Autodesk Fusion 360 part; units mm, degrees
sketch "Control Panel Top" plane through (0, 0, 0) normal (0, 0, 1) x (1, 0, 0)
  line L0 (0, 0) -> (270, 0)
  line L1 (270, 0) -> (270, 86.085)
  line L2 (270, 86.085) -> (0, 86.085)
  line L3 (0, 86.085) -> (0, 0)
  dimension "d6" = 270
  dimension "d7" = 86.085
extrude "Extrude1" add sketch "Control Panel Top" along normal blind 6
sketch "Button Layout" plane through (0, 0, 6) normal (0, 0, 1) x (-1, 0, 0)
  line L0 (0, -86.085) -> (0, 0)
  line L1 (0, 0) -> (-270, 0)
  line L2 (-270, 0) -> (-270, -86.085)
  line L3 (-270, -86.085) -> (0, -86.085)
  circle A0 centre (-90, -43) radius 15
  circle A1 centre (-140, -43) radius 15
  circle A2 centre (-40, -43) radius 15
  dimension "d12" = 30
  dimension "d13" = 30
  dimension "d14" = 30
  dimension "d17" = 40
  dimension "d20" = 50
  dimension "d21" = 43
  dimension "d22" = 43
  dimension "d23" = 43
  dimension "d24" = 50
extrude "Extrude2" cut sketch "Button Layout" against normal blind 6 contours A0 | A1
extrude "Extrude3" cut sketch "Button Layout" against normal blind 6 contours A2
equation "MDFThickness = 6 mm"
equation "d2 = MDFThickness"
equation "controlPanelTopLength = 75 mm"
equation "controlPanelTopWidth = 250 mm"
equation "arcadeButtonDiameter = 30 mm"
equation "d12 = arcadeButtonDiameter"
equation "d13 = arcadeButtonDiameter"
equation "d14 = arcadeButtonDiameter"
equation "d21 = ( 86 / 2 ) * 1 mm"
equation "d22 = ( 86 / 2 ) * 1 mm"
equation "d23 = ( 86 / 2 ) * 1 mm"
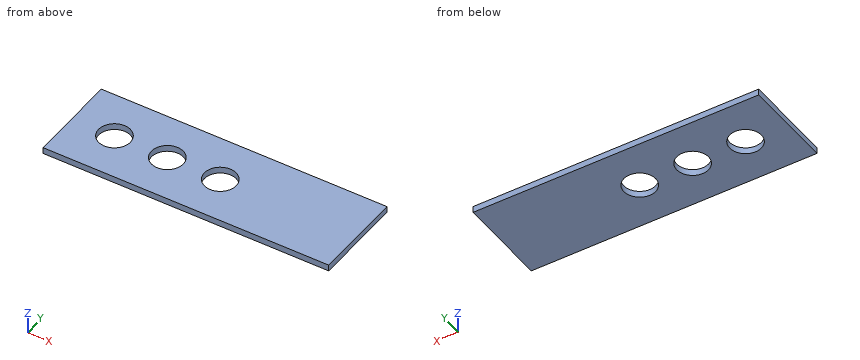
Can you work these out from the model? Positions are in its coordinate system, mm. Coordinates: 2 decimals unless noted, no trailing zeros. Write each loop counter-clockwise with the first axis right and the second up, starting at its lowest first coordinate (ties: lowest second). Pieces come first, ordered by that corner, then holes. Notation, with made-up numbers: (-1.5, -9.75) -> (6.5, -9.75) arc R33 ccw to (6.5, 28.25) -> close; hole circle Ø6 at (26.25, 66.5). An arc over 180 degrees is marked (long way). Write each question's results on one line, items separated by ' | '. Start each with the question number.
Item 1: If we section it at C-C, the plane z = 1.7: Write out the boundary of the cut face in (x, y) (3 decimals), and give its area (3 significant figures).
Item 2: If we section it at D-D, the plane y = 31: Write out the boundary of the cut face in (x, z), and give its area (3 significant figures).
Item 3: If we section it at B-B, the plane x = 140: Write out the boundary of the cut face in (y, z) (3 decimals).
Item 4: If we section it at A-A, the plane y = 43: Write out the boundary of the cut face in (x, z), and give its area (3 significant figures).
Item 5: Please list where these lines run through material, in increasing order: probe 1 along X at (y, z) = (43, 3.3); probe 2 along Y at (x, z) = (90, 2.4) (3 decimals); probe 3 along Y at (x, z) = (28, 1.45) (3 decimals).
Answer block:
1) outline: (0, 0) -> (270, 0) -> (270, 86.085) -> (0, 86.085) -> close; hole circle Ø30 at (40, 43); hole circle Ø30 at (90, 43); hole circle Ø30 at (140, 43) | area: 21,100 mm²
2) outline: (0, 0) -> (31, 0) -> (31, 6) -> (0, 6) -> close; (49, 0) -> (81, 0) -> (81, 6) -> (49, 6) -> close; (99, 0) -> (131, 0) -> (131, 6) -> (99, 6) -> close; (149, 0) -> (270, 0) -> (270, 6) -> (149, 6) -> close | area: 1,300 mm²
3) outline: (0, 0) -> (28, 0) -> (28, 6) -> (0, 6) -> close; (58, 0) -> (86.085, 0) -> (86.085, 6) -> (58, 6) -> close
4) outline: (0, 0) -> (25, 0) -> (25, 6) -> (0, 6) -> close; (55, 0) -> (75, 0) -> (75, 6) -> (55, 6) -> close; (105, 0) -> (125, 0) -> (125, 6) -> (105, 6) -> close; (155, 0) -> (270, 0) -> (270, 6) -> (155, 6) -> close | area: 1,080 mm²
5) probe 1: 0 to 25, 55 to 75, 105 to 125, 155 to 270 | probe 2: 0 to 28, 58 to 86.085 | probe 3: 0 to 34, 52 to 86.085
